Input: part model. Units: mm. Frame: model coordinates. A direction names the side the tool comes from. Round coordinates to 2 decimals unless told otherwise and drop trailing zeros. Write each loop counter-clockwise with the first axis right and the second up, starting at its lowest first coordinate (ties: lowest second). Pieces come first, ordered by that corner, then holes. Notation, with made-up numbers: (56, -14.5) - (84, -14.5) arc R29 cw to (84, 6.5) - close; hole circle Ø8 at (50.5, 72). An arc over 180 degrees is marked (long way). Use one line per item in the form item = value.
```python
from build123d import *

# Parameters (mm, degrees)
SKETCH1_W                               = 482.6
SKETCH1_H                               = 406.4
BOSS_EXTRUDE1_DEPTH                     = 26.416
SKETCH3_R                               = 1.27
SKETCH3_R_2                             = 5.25
CUT_EXTRUDE2_DEPTH                      = 27.416
CBORE_FOR_M10_HEX_HEAD_BOLT1_AT_2_COUNT = 2
CBORE_FOR_M10_HEX_HEAD_BOLT1_AT_2_PITCH = 55.7
CBORE_FOR_M10_HEX_HEAD_BOLT1_AT_3_COUNT = 2
CBORE_FOR_M10_HEX_HEAD_BOLT1_AT_3_PITCH = 96.475229982
CBORE_FOR_M10_HEX_HEAD_BOLT1_AT_4_COUNT = 2
CBORE_FOR_M10_HEX_HEAD_BOLT1_AT_4_PITCH = 111.4
CBORE_FOR_M10_HEX_HEAD_BOLT1_AT_5_COUNT = 2
CBORE_FOR_M10_HEX_HEAD_BOLT1_AT_5_PITCH = 96.475229982
CBORE_FOR_M10_HEX_HEAD_BOLT1_AT_6_COUNT = 2
CBORE_FOR_M10_HEX_HEAD_BOLT1_AT_6_PITCH = 55.7
TAP_DRILL_FOR_M10_HELICOIL1_D           = 10.5


with BuildPart() as part:
    # Sketch1 → Boss-Extrude1 (new body)
    with BuildSketch(Plane(origin=(0, 0, 0), x_dir=(1, 0, 0), z_dir=(0, 1, 0))):
        Rectangle(SKETCH1_W, SKETCH1_H)
    extrude(amount=BOSS_EXTRUDE1_DEPTH)

    # Sketch3 → Cut-Extrude2 (cut, through all)
    with BuildSketch(Plane(origin=(0, 26.416, 0), x_dir=(1, 0, 0), z_dir=(0, 1, 0))):
        with Locations((-185.152559706, -80.01)):
            Circle(SKETCH3_R)
        with Locations((-159.68726, -80.01)):
            Circle(SKETCH3_R)
        with Locations((-185.152559706, 80.01)):
            Circle(SKETCH3_R)
        with Locations((-159.68726, 80.01)):
            Circle(SKETCH3_R)
        with Locations((159.68726, -80.01)):
            Circle(SKETCH3_R)
        with Locations((185.152559706, -80.01)):
            Circle(SKETCH3_R)
        with Locations((185.152559706, 80.01)):
            Circle(SKETCH3_R)
        with Locations((159.68726, 80.01)):
            Circle(SKETCH3_R)
        with Locations((55.7, 0)):
            Circle(SKETCH3_R_2)
        with Locations((27.85, -48.237614991)):
            Circle(SKETCH3_R_2)
        with Locations((-27.85, -48.237614991)):
            Circle(SKETCH3_R_2)
        with Locations((-55.7, 0)):
            Circle(SKETCH3_R_2)
        with Locations((-27.85, 48.237614991)):
            Circle(SKETCH3_R_2)
        with Locations((27.85, 48.237614991)):
            Circle(SKETCH3_R_2)
    extrude(amount=-CUT_EXTRUDE2_DEPTH, mode=Mode.SUBTRACT)

    # Sketch11 → CBORE for M10 Hex Head Bolt1 (revolve, cut)
    with BuildSketch(Plane(origin=(27.85, 26.416, -48.237614991), x_dir=(0, 0, 1), z_dir=(1, 0, 0))):
        Polygon((0, 0), (0, 26.416), (6, 26.416), (6, 7.5), (10.74, 7.5), (10.74, 0.025), (10.765, 0), align=None)
    cbore_for_m10_hex_head_bolt1 = revolve(axis=Axis((27.85, 32.766, -48.237614991), (0, -1, 0)), mode=Mode.SUBTRACT)

    # CBORE for M10 Hex Head Bolt1 at 2: CBORE for M10 Hex Head Bolt1 ×2
    with Locations(*[Vector(0.5, 0, 0.866025404) * (i * CBORE_FOR_M10_HEX_HEAD_BOLT1_AT_2_PITCH) for i in range(1, CBORE_FOR_M10_HEX_HEAD_BOLT1_AT_2_COUNT)]):
        add(cbore_for_m10_hex_head_bolt1, mode=Mode.SUBTRACT)

    # CBORE for M10 Hex Head Bolt1 at 3: CBORE for M10 Hex Head Bolt1 ×2
    with Locations(*[(0, 0, i * CBORE_FOR_M10_HEX_HEAD_BOLT1_AT_3_PITCH) for i in range(1, CBORE_FOR_M10_HEX_HEAD_BOLT1_AT_3_COUNT)]):
        add(cbore_for_m10_hex_head_bolt1, mode=Mode.SUBTRACT)

    # CBORE for M10 Hex Head Bolt1 at 4: CBORE for M10 Hex Head Bolt1 ×2
    with Locations(*[Vector(-0.5, 0, 0.866025404) * (i * CBORE_FOR_M10_HEX_HEAD_BOLT1_AT_4_PITCH) for i in range(1, CBORE_FOR_M10_HEX_HEAD_BOLT1_AT_4_COUNT)]):
        add(cbore_for_m10_hex_head_bolt1, mode=Mode.SUBTRACT)

    # CBORE for M10 Hex Head Bolt1 at 5: CBORE for M10 Hex Head Bolt1 ×2
    with Locations(*[Vector(-0.866025404, 0, 0.5) * (i * CBORE_FOR_M10_HEX_HEAD_BOLT1_AT_5_PITCH) for i in range(1, CBORE_FOR_M10_HEX_HEAD_BOLT1_AT_5_COUNT)]):
        add(cbore_for_m10_hex_head_bolt1, mode=Mode.SUBTRACT)

    # CBORE for M10 Hex Head Bolt1 at 6: CBORE for M10 Hex Head Bolt1 ×2
    with Locations(*[(-i * CBORE_FOR_M10_HEX_HEAD_BOLT1_AT_6_PITCH, 0, 0) for i in range(1, CBORE_FOR_M10_HEX_HEAD_BOLT1_AT_6_COUNT)]):
        add(cbore_for_m10_hex_head_bolt1, mode=Mode.SUBTRACT)

    # Tap Drill for M10 Helicoil1 (through all)
    with Locations(Plane(origin=(0, 26.416, 0), x_dir=(1, 0, 0), z_dir=(0, 1, 0))):
        with Locations((-185.152559706, -80.01), (-159.68726, -80.01), (-185.152559706, 80.01), (-159.68726, 80.01), (185.152559706, 80.01), (159.68726, 80.01), (185.152559706, -80.01), (159.68726, -80.01)):
            Hole(TAP_DRILL_FOR_M10_HELICOIL1_D / 2)


solid = part.part
```
(1) Access query for faces 1 (the face through (-154.442, 13.023, -80.241)), 2 (the face through (65.228, 22.706, 4.956)). Directions: +Z, -Z, +X, -X, +Y, -Y. A direction counts if a zero-diameter tool reaches every point of the face in a straight line with its end or side. Return the directions, or none.
Derived:
face_1 = +Y, -Y
face_2 = +Y
(2) First-contact query: pin 1 Ø24.5 at (x, z) = (-55.7, 0) entering from +Y. Flat tip, straight axial feed; report the tip coordinate or a pass-through.
Derived:
pin_1 = 26.42
(3) Cut plane C-C on z = -80.01. Output: boundary loops of the cut face in (x, y), then the cut area to 3 significant figures.
Derived:
outline = (-241.3, 0) - (-190.4, 0) - (-190.4, 26.42) - (-241.3, 26.42) - close; (-179.9, 0) - (-164.94, 0) - (-164.94, 26.42) - (-179.9, 26.42) - close; (-154.44, 0) - (154.44, 0) - (154.44, 26.42) - (-154.44, 26.42) - close; (164.94, 0) - (179.9, 0) - (179.9, 26.42) - (164.94, 26.42) - close; (190.4, 0) - (241.3, 0) - (241.3, 26.42) - (190.4, 26.42) - close
area = 11,600 mm^2
(4) Draft query along Z for faces 3 (the face through (-3, 13, -203.2)), 4 (the face through (-241.3, 13, 3)), 5 (the face through (-45.215, 22.706, -2.328)). Return one class per face: released by +Z, released by -Z, zero draft, split by the parting line, or undercut.
Derived:
face_3 = released by -Z
face_4 = zero draft
face_5 = undercut
(5) Cut plane B-B on z = 0. Output: boundary loops of the cut face in (x, y) (3 decimals), then the cut area to 3 significant figures.
Derived:
outline = (-241.3, 0) - (-61.7, 0) - (-61.7, 18.916) - (-66.44, 18.916) - (-66.44, 26.391) - (-66.465, 26.416) - (-241.3, 26.416) - close; (-49.7, 0) - (49.7, 0) - (49.7, 18.916) - (44.96, 18.916) - (44.96, 26.391) - (44.935, 26.416) - (-44.935, 26.416) - (-44.96, 26.391) - (-44.96, 18.916) - (-49.7, 18.916) - close; (61.7, 0) - (241.3, 0) - (241.3, 26.416) - (66.465, 26.416) - (66.44, 26.391) - (66.44, 18.916) - (61.7, 18.916) - close
area = 12,000 mm^2
(6) Material intervals for L1, parallel to Z at x = 27.85, y = 24; L2, parallel to X at y = 23.25, z = 0; L3, parallel to Z at x = -27.85, y = 9.25, sorted ascending.
Derived:
L1 = -203.2 to -58.98, -37.5 to 37.5, 58.98 to 203.2
L2 = -241.3 to -66.44, -44.96 to 44.96, 66.44 to 241.3
L3 = -203.2 to -54.24, -42.24 to 42.24, 54.24 to 203.2
(7) Cut plane A-A on x = 27.85. Count the separate pieces of the cut face and the enclosed holes in it, then the cut area to 3 significant figures.
Derived:
separate_pieces = 3
enclosed_holes = 0
area = 9,960 mm^2
